Design review of the part built by this model. Coordinates are the model's own, in mm. A direction names the side the tool comes from. Coordinates: 2 decimals unless noted, no trailing zeros. Loops run counter-clockwise (first coordinate to the right, second up) from the corner with the lowest first, then second, coordinate; pieces in that order, holes last. Notation, with made-up numbers: (67.25, -3) -> (109.25, -3) arc R21 cw to (109.25, 10) -> close; hole circle Ø5 at (-40, 52.5). An arc over 180 degrees is marked (long way). Use a Markdown table: item, result. Add a question column.
Q1. For probe 1 along Z at (x, y) = (-31.5, -36.25); probe 2 along Y at (x, z) = (0, -1.25); probe 3 along Y at (x, z) = (35, 5), list the stretches that pass through material, from the lowest coordinate up.
Q2. Take a section at A-A on x = 0. Write out the cut boundary in (y, z).
Q3. Draft analysis for pull direction X (two halves, no side actions). For faces 1 (the face through (30, -32, -3)), 2 (the face through (2.285, 3.584, -0.084)), 3 (the face through (-12.5, -13, 0)), 4 (the face through (12.5, -14, 0)), state which applies: pulls with the +X half, pulls with the -X half, needs draft (parallel to the pull), parting line crosses it, or undercut.
Q4. Clearance check with flat-ended pins moving along their axes: pin 1 Ø5 at (y, z) = (-4, -3) entering from +X; pin 2 Ø6 at (y, z) = (-7, 0) entering from -X; pin 3 Ø3.5 at (x, z) = (34, 2.5) entering from +Y. State where each tip first meets the part, or that it passes through.
Q5. Take a section at B-B on y = 3. Write out the cut boundary in (x, z).
Q6. Take a section at C-C on x = -19. Write out the cut boundary in (y, z).
Q7. Take a section at D-D on y = -18. Write out the cut boundary in (x, z).
Q8. For faces 5 (the face through (-30, -36, -2.5)), 6 (the face through (13.93, -30.5, 0.08)), list the 3-axis set-ups (+Z, -Z, +X, -X, +Y, -Y) from which the entire face can be reached by the end or side of a thin tool; tool diameter is ignored.
from build123d import *

# Parameters (mm, degrees)
BOSS_EXTRUDE1_DEPTH      = 6
BOSS_EXTRUDE1_DEPTH_BACK = 6
SKETCH1_R                = 12.5
SKETCH1_R_2              = 4.25
CUT_EXTRUDE1_DEPTH       = 59.330952332
FILLET1_R                = 5


with BuildPart() as part:
    # Sketch1 → Boss-Extrude1 (new, two sides: drawn at the far end of the back side and taken through both)
    # profile 1 of 2: a face of its own
    with BuildSketch(Plane.XY.offset(-BOSS_EXTRUDE1_DEPTH_BACK)):
        Circle(SKETCH1_R)
        Circle(SKETCH1_R_2, mode=Mode.SUBTRACT)
    # profile 2 of 2: a face of its own
    with BuildSketch(Plane.XY.offset(-BOSS_EXTRUDE1_DEPTH_BACK)):
        with BuildLine():
            Line((-42.5, -32), (-42.5, -39.5))
            Line((-42.5, -39.5), (42.5, -39.5))
            Line((42.5, -39.5), (42.5, -32))
            Line((42.5, -32), (12.5, -32))
            Line((12.5, -32), (12.5, 0))
            ThreePointArc((12.5, 0), (0, -12.5), (-12.5, 0))
            Line((-12.5, 0), (-12.5, -32))
            Line((-12.5, -32), (-42.5, -32))
        make_face()
    extrude(amount=BOSS_EXTRUDE1_DEPTH + BOSS_EXTRUDE1_DEPTH_BACK)

    # Sketch4 → Cut-Extrude1 (cut, through all)
    with BuildSketch(Plane(origin=(0, 0, 0), x_dir=(1, 0, 0), z_dir=(0, 1, 0))):
        with BuildLine():
            ThreePointArc((31.025, -2.454460226), (34, 0), (31.025, 2.454460226))
            ThreePointArc((31.025, 2.454460226), (31.035274533, 2.477251617), (31.045643943, 2.5))
            Line((31.045643943, 2.5), (28, 2.5))
            ThreePointArc((28, 2.5), (25.5, 0), (28, -2.5))
            Line((28, -2.5), (31.045643943, -2.5))
            ThreePointArc((31.045643943, -2.5), (31.035274533, -2.477251617), (31.025, -2.454460226))
        make_face()
        with BuildLine():
            ThreePointArc((42.5, 0), (40.742640687, -4.242640687), (36.5, -6))
            Line((36.5, -6), (42.5, -6))
            Line((42.5, -6), (42.5, 0))
        make_face()
        with BuildLine():
            Line((-42.5, -6), (-36.5, -6))
            ThreePointArc((-36.5, -6), (-40.742640687, -4.242640687), (-42.5, 0))
            Line((-42.5, 0), (-42.5, -6))
        make_face()
        with BuildLine():
            ThreePointArc((36.5, 6), (40.742640687, 4.242640687), (42.5, 0))
            Line((42.5, 0), (42.5, 6))
            Line((42.5, 6), (36.5, 6))
        make_face()
        with BuildLine():
            Line((-42.5, 6), (-42.5, 0))
            ThreePointArc((-42.5, 0), (-40.742640668, 4.242640706), (-36.499999946, 6))
            Line((-36.499999946, 6), (-42.5, 6))
        make_face()
        with BuildLine():
            ThreePointArc((-31.045643943, 2.5), (-31.035274533, 2.477251617), (-31.025, 2.454460226))
            ThreePointArc((-31.025, 2.454460226), (-34, 0), (-31.025, -2.454460226))
            ThreePointArc((-31.025, -2.454460226), (-31.035274533, -2.477251617), (-31.045643943, -2.5))
            Line((-31.045643943, -2.5), (-28, -2.5))
            ThreePointArc((-28, -2.5), (-25.5, 0), (-28, 2.5))
            Line((-28, 2.5), (-31.045643943, 2.5))
        make_face()
    extrude(amount=-CUT_EXTRUDE1_DEPTH, mode=Mode.SUBTRACT)

    # Fillet1
    fillet1_edges = [part.edges().sort_by_distance(p)[0] for p in [
        (12.5, -32, 0),
        (-12.5, -32, 0),
    ]]
    fillet(fillet1_edges, radius=FILLET1_R)


solid = part.part
Answer list:
| question | item | result |
|---|---|---|
| 1 | probe 1 | -6 to -2.5, 2.5 to 6 |
| 1 | probe 2 | -39.5 to -4.25, 4.25 to 12.5 |
| 1 | probe 3 | -39.5 to -32 |
| 2 | outline | (-39.5, -6) -> (-4.25, -6) -> (-4.25, 6) -> (-39.5, 6) -> close; (4.25, -6) -> (12.5, -6) -> (12.5, 6) -> (4.25, 6) -> close |
| 3 | face 1 | needs draft |
| 3 | face 2 | undercut |
| 3 | face 3 | pulls with the -X half |
| 3 | face 4 | pulls with the +X half |
| 4 | pin 1 | x = 12.5 |
| 4 | pin 2 | x = -12.5 |
| 4 | pin 3 | y = -32 |
| 5 | outline | (-12.13, -6) -> (-3.01, -6) -> (-3.01, 6) -> (-12.13, 6) -> close; (3.01, -6) -> (12.13, -6) -> (12.13, 6) -> (3.01, 6) -> close |
| 6 | outline | (-39.5, -6) -> (-32, -6) -> (-32, 6) -> (-39.5, 6) -> close |
| 7 | outline | (-12.5, -6) -> (12.5, -6) -> (12.5, 6) -> (-12.5, 6) -> close |
| 8 | face 5 | +Y, -Y |
| 8 | face 6 | +Z, -Z, +X, +Y |
